Verification items for the finished model (mm, model axes). Face numbers are marked on the shaded views. A direction names the side the tool comes from. Round coordinates to 2 decimals unless told otherwise and drop trailing zeros. Order: outer loops, then holes, each group sorted by start corner. A loop starts at its lowest first (then second) coordinate and runs counter-clockwise, first axis right, second up. Notation, with made-up numbers: (23.25, 22.5) -> (36.25, 22.5) arc R27 ccw to (36.25, 54.5) -> close; hole circle Ø4 at (71.5, -3). An arc over 180 degrees is marked (long way). Put each result on its own line as item: value.
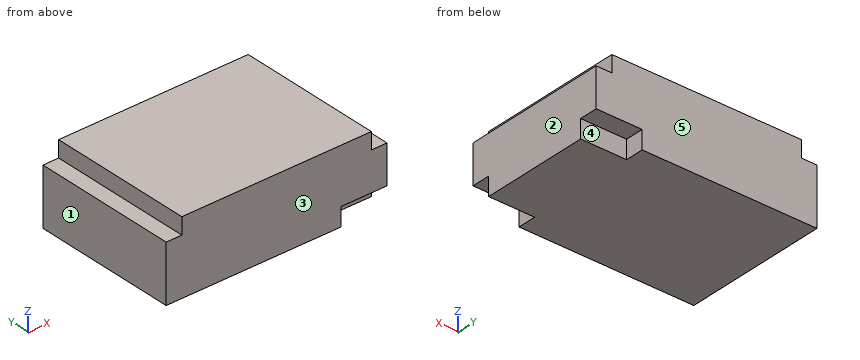
from build123d import *

# Parameters (mm, degrees)
SKETCH_W        = 120
SKETCH_H        = 79
PAD_DEPTH       = 31
SKETCH001_W     = 103
SKETCH001_H     = 79
PAD001_DEPTH    = 9
SKETCH003_W     = 25
SKETCH003_H     = 10
POCKET_DEPTH    = 10
SKETCH004_W     = 25
SKETCH004_H     = 10
POCKET001_DEPTH = 10


with BuildPart() as part:
    # Sketch → Pad (new body)
    with BuildSketch(Plane.XY):
        Rectangle(SKETCH_W, SKETCH_H)
    extrude(amount=PAD_DEPTH)

    # Sketch001 → Pad001 (join)
    with BuildSketch(Plane.XY.offset(31)):
        Rectangle(SKETCH001_W, SKETCH001_H)
    extrude(amount=PAD001_DEPTH)

    # Sketch003 (on Face4 of Pad001) → Pocket (cut)
    with BuildSketch(Plane(origin=(0, 0, 0), x_dir=(1, 0, 0), z_dir=(0, 0, -1))):
        with Locations((47.5, -34.5)):
            Rectangle(SKETCH003_W, SKETCH003_H)
    extrude(amount=-POCKET_DEPTH, mode=Mode.SUBTRACT)

    # Sketch004 (on Face2 of Pocket) → Pocket001 (cut)
    with BuildSketch(Plane(origin=(0, 0, 0), x_dir=(1, 0, 0), z_dir=(0, 0, -1))):
        with Locations((47.5, 34.5)):
            Rectangle(SKETCH004_W, SKETCH004_H)
    extrude(amount=-POCKET001_DEPTH, mode=Mode.SUBTRACT)


solid = part.part
Item 1: Gauge pin test, flat ends, axial feed: pin 1 Ø1.5 at (x, y) = (-33, -6) entering from -Z; pin 2 Ø9.5 at (x, y) = (56.5, 16) entering from +Z; pin 3 Ø5 at (x, z) = (46, 3) entering from +Y; pin 4 Ø11 at (x, z) = (52, 4) entering from -Y. Record the tip position at first contact, or that the pin passes through.
Check sheet entries:
pin 1: stops at z = 0
pin 2: stops at z = 31
pin 3: stops at y = 29.5
pin 4: stops at y = -29.5
Item 2: Section check A-A on y = -21. Record the boundary of the cut face in (x, z).
Check sheet entries:
outline: (-60, 0) -> (60, 0) -> (60, 31) -> (51.5, 31) -> (51.5, 40) -> (-51.5, 40) -> (-51.5, 31) -> (-60, 31) -> close
Item 3: Release check for a two-part mould opening along X. For the marked faces 1, 2 and 3 record: +X half, -X half, draft (parallel to the pull), parting line (faces both ways), or undercut.
Check sheet entries:
face 1: -X half
face 2: +X half
face 3: draft
Item 4: Section check B-B on x = 45.5. Record the boundary of the cut face in (y, z).
Check sheet entries:
outline: (-39.5, 10) -> (-29.5, 10) -> (-29.5, 0) -> (29.5, 0) -> (29.5, 10) -> (39.5, 10) -> (39.5, 40) -> (-39.5, 40) -> close
Item 5: Material ranges on L1, parallel to X at y = -28, z = 35; L2, parallel to X at y = -34, z = 9, recorded low to high. Write a range as [from, to].
Check sheet entries:
L1: x = [-51.5, 51.5]
L2: x = [-60, 35]
Item 6: Tool access check on the marked faces 4 and 5. Record the directions out of +Z, -Z, +X, -X, +Y, -Y that give a thin tool (end or side, any length) a straight path to the whole face; none if there is none.
Check sheet entries:
face 4: -Z, +X, +Y
face 5: +Z, -Z, +X, -X, +Y
Item 7: Section check C-C on x = -53. Record the boundary of the cut face in (y, z).
Check sheet entries:
outline: (-39.5, 0) -> (39.5, 0) -> (39.5, 31) -> (-39.5, 31) -> close
